Drawing for the job (mm, zero at the part's lowest x, y, z). A direction names the side the tool comes from. Round coordinates to 2 decimals unless told otherwise and drop trailing zeros. Loops run counter-clockwise (first coordinate to the right, second up) from the corner with the lowest first, then second, coordinate; pieces in that order, holes last. Notation, with made-up numbers: M 51.25,15 L 67.25,15 A30 cw 67.25,54 Z; hole C 65.25,-18.75 d3. An arc over 180 degrees is marked long. Use a Markdown table: item, result. Add a question column.
Q1. Cut at D-D (x = 4). Give the cut face in (y, z).
Q2. Cut at C-C (z = 7.5). Give the cut face in (x, y).
Q3. Tool access for the marked faces 4, 5, 6 and 7: list every direction of +Z, -Z, +X, -X, +Y, -Y with a clear straight run to the whole face (end or side of a thin tool).
Q4. Mould opens along X. For the marked faces 1, 2 and 3 say: +X half, -X half, draft (parallel to the pull), parting line (faces both ways), or undercut.
Q5. Pin check, flat tips, straight feed: pin 1 (7.5 mm diameter, centred on y = 6, z = 10, fed in from +X); pin 2 (5.5 mm diameter, centred on x = 4, z = 7.5, fed in from -Y); pin 3 (5 mm diameter, centred on y = 5.5, z = 6.5, fed in from -X). Stop position of each tip, or through.
Q6. Probe line 1 (X direction, y = 23.75, z = 7.5); line 2 (X direction, y = 7.5, z = 0.75); line 3 (Y direction, x = 48, z = 11.75). List the from-to ranges inside material, lowest first. Write a range as from..to.
Q7. Cut at A-A (y = 22.75). Give the cut face in (x, z).
Q8. Cut at B-B (y = 11.5). Give the cut face in (x, z).
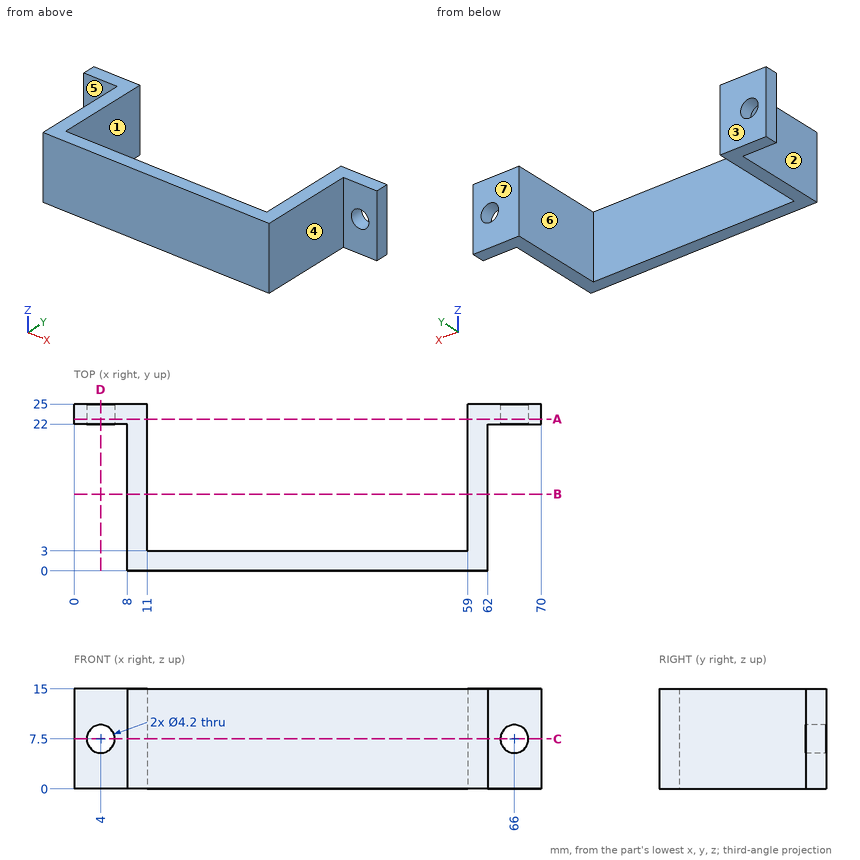
Checked values:
| question | item | result |
|---|---|---|
| 1 | outline | M 22,0 L 25,0 L 25,5.4 L 22,5.4 Z; M 22,9.6 L 25,9.6 L 25,15 L 22,15 Z |
| 2 | outline | M 0,22 L 1.9,22 L 1.9,25 L 0,25 Z; M 6.1,22 L 8,22 L 8,0 L 62,0 L 62,22 L 63.9,22 L 63.9,25 L 59,25 L 59,3 L 11,3 L 11,25 L 6.1,25 Z; M 68.1,22 L 70,22 L 70,25 L 68.1,25 Z |
| 3 | face 4 | +Z, -Z, +X, -Y |
| 3 | face 5 | +Z, -Z, -X, -Y |
| 3 | face 6 | +Z, -Z, +Y |
| 3 | face 7 | +Z, -Z, +X, -X, +Y |
| 4 | face 1 | undercut |
| 4 | face 2 | -X half |
| 4 | face 3 | draft |
| 5 | pin 1 | stops at x = 62 |
| 5 | pin 2 | stops at y = 22 |
| 5 | pin 3 | stops at x = 8 |
| 6 | line 1 | x = 0..1.9, 6.1..11, 59..63.9, 68.1..70 |
| 6 | line 2 | x = 8..11, 59..62 |
| 6 | line 3 | y = 0..3 |
| 7 | outline | M 0,0 L 11,0 L 11,15 L 0,15 Z; M 59,0 L 70,0 L 70,15 L 59,15 Z; hole C 4,7.5 d4.2; hole C 66,7.5 d4.2 |
| 8 | outline | M 8,0 L 11,0 L 11,15 L 8,15 Z; M 59,0 L 62,0 L 62,15 L 59,15 Z |
